Check sheet for the modelled part. Datum: model origin and axes. Units: mm. A direction names the side the tool comes from. Round coordinates to 2 decimals unless told otherwise and drop trailing zeros. Loops run counter-clockwise (first coordinate to the right, second up) from the corner with the lowest first, then second, coordinate; pieces in that order, holes last. Notation, with made-up numbers: M 14,-10 L 55,-10 A9 cw 55,-6 Z; hole C -36.75,-10 d2. An arc over 180 degrees is marked long. One line per question, with ' | ' between items. Start each with the question number.
(1) Section check C-C (z = -23). Record the boundary of the cut face in (x, y), and give its area (3 significant figures).
(2) Section check D-D (y = 37.5). Record the boundary of the cut face in (x, z).
(3) Tool access check on faces 1 (the face through (56, 3, -14)), 2 (the face through (15, 13, -28)), 3 (the face through (34, 0.9, -34)), 4 (the face through (21, 21, -14)), 5 (the face through (59, 1.5, -14)). Record the directions out of +Z, -Z, +X, -X, +Y, -Y that give a thin tool (end or side, any length) a straight path to the whole face; none if there is none.
(4) Draft check along X on faces 6 (the face through (15, 13, 0)), 7 (the face through (0, 2.2, -14.3)), 8 (the face through (66, 4, -14)). Enter one of: +X half, -X half, draft (parallel to the pull), parting line (faces both ways), or undercut.
(5) Go/stop test with flat-tipped pins: P1, Ø8, axis at x = 7.5, y = 11.5, coming from the -Z side; P2, Ø1.5, axis at x = 13, z = -9.5, coming from the +Y side; P3, Ø2, axis at x = 59.5, z = -14, coming from the -Y side. Record where each tip stops, or that it passes through.
(6) Section check B-B (x = 28.5). Record the boundary of the cut face in (y, z).
(7) Thickness scan on probe 1 along Z at (x, y) = (15.5, 16); probe 2 along X at (y, z) = (9.5, -6); probe 3 along Y at (x, z) = (33, -34). Record the ranges inside material, lowest first. Write a range as [from, to].
(8) Section check A-A (y = 21.5). Record the boundary of the cut face in (x, z).
```python
from build123d import *

# Parameters (mm, degrees)
SKETCH1_W           = 21
SKETCH1_H           = 28
BOSS_EXTRUDE1_DEPTH = 3
SKETCH2_W           = 21
SKETCH2_H           = 28
BOSS_EXTRUDE2_DEPTH = 37
CUT_EXTRUDE1_REACH  = 55.151
SHELL1_T            = -1
BOSS_EXTRUDE3_DEPTH = 33.5
SKETCH9_W           = 21
SKETCH9_H           = 28
CUT_EXTRUDE2_DEPTH  = 2
SKETCH10_R          = 1
BOSS_EXTRUDE4_DEPTH = 0.5
CUT_EXTRUDE3_REACH  = 59.099
SKETCH11_W          = 2.558101437
SKETCH11_H          = 1.124051106
MIRROR5_START       = -28
MIRROR5_DEPTH       = 28
MIRROR5_START_2     = 1.5
MIRROR5_2_OUTLINE_R = 1
MIRROR5_2_DEPTH     = 0.5
SHELL3_START        = -27
SHELL3_DEPTH        = 26


# Read off the part's stored shape, not the designer's step: Mirror5, Shell3
with BuildPart() as part:
    # Sketch1 → Boss-Extrude1 (new body)
    with BuildSketch(Plane(origin=(0, 0, 0), x_dir=(1, 0, 0), z_dir=(0, 1, 0))):
        with Locations((10.5, 14)):
            Rectangle(SKETCH1_W, SKETCH1_H)
    extrude(amount=BOSS_EXTRUDE1_DEPTH)

    # Sketch2 → Boss-Extrude2 (add)
    with BuildSketch(Plane(origin=(0, 3, 0), x_dir=(1, 0, 0), z_dir=(0, 1, 0))):
        with Locations((10.5, 14)):
            Rectangle(SKETCH2_W, SKETCH2_H)
    extrude(amount=BOSS_EXTRUDE2_DEPTH)

    # Sketch3 → Cut-Extrude1 (cut, up to next)
    with BuildSketch(Plane.XY, mode=Mode.PRIVATE) as cut_extrude1_sk1:
        Polygon((0, 3), (21, 40), (0, 40), align=None)
    cut_extrude1_tool1 = extrude(cut_extrude1_sk1.sketch, amount=-CUT_EXTRUDE1_REACH, mode=Mode.PRIVATE) & part.part
    add(cut_extrude1_tool1.solids().sort_by_distance((7, 27.666667, 0))[0], mode=Mode.SUBTRACT)

    # Shell1
    shell1_openings = [part.faces().sort_by_distance(p)[0] for p in [
        (10.5, 21.5, -14),
    ]]
    offset(amount=SHELL1_T, openings=shell1_openings, kind=Kind.INTERSECTION)

    # Sketch7 → Boss-Extrude3 (add)
    with BuildSketch(Plane(origin=(0, 0, 0), x_dir=(0, 0, -1), z_dir=(1, 0, 0))):
        Polygon((34, -0.1), (32.967936428, -0.1), (32.967936428, 0.9), (34.5, 0.9), (34.5, 2), (29.5, 2), (-1.5, 2), (-6.5, 2), (-6.5, 0.9), (-4.967936428, 0.9), (-4.967936428, -0.1), (-6, -0.1), (-7.5, -0.1), (-7.5, 3), (-1.5, 3), (29.5, 3), (35.5, 3), (35.5, -0.1), align=None)
    boss_extrude3 = extrude(amount=BOSS_EXTRUDE3_DEPTH)

    # Sketch9 → Cut-Extrude2 (cut)
    with BuildSketch(Plane.XZ):
        with Locations((10.5, -14)):
            Rectangle(SKETCH9_W, SKETCH9_H)
    extrude(amount=-CUT_EXTRUDE2_DEPTH, mode=Mode.SUBTRACT)

    # Sketch10 → Boss-Extrude4 (add)
    with BuildSketch(Plane.XZ.offset(-2)):
        with Locations(Location((8, -14, 0), (0, 0, 90))):
            Circle(SKETCH10_R)
    extrude(amount=BOSS_EXTRUDE4_DEPTH)

    # Sketch11 → Cut-Extrude3 (cut, up to next)
    with BuildSketch(Plane.ZY.offset(-20), mode=Mode.PRIVATE) as cut_extrude3_sk1:
        with Locations((-15.279050719, 10.379008518)):
            Rectangle(SKETCH11_W, SKETCH11_H)
    cut_extrude3_tool1 = extrude(cut_extrude3_sk1.sketch, amount=-CUT_EXTRUDE3_REACH, mode=Mode.PRIVATE) & part.part
    cut_extrude3 = cut_extrude3_tool1.solids().sort_by_distance((20, 10.379009, -15.279051))[0]
    add(cut_extrude3, mode=Mode.SUBTRACT)

    # Mirror4: Boss-Extrude3 across plane
    add(boss_extrude3.mirror(Plane(origin=(33.5, 0, 0), x_dir=(0, 0, 1), z_dir=(1, 0, 0))))

    # Mirror5 outline → Mirror5 (add)
    with BuildSketch(Plane.XY.offset(MIRROR5_START)):
        Polygon((67, 3), (46, 40), (46, 3), align=None)
    extrude(amount=MIRROR5_DEPTH)

    # Mirror5 2 outline → Mirror5 2 (add)
    with BuildSketch(Plane(origin=(0, 0, 0), x_dir=(1, 0, 0), z_dir=(0, 1, 0)).offset(MIRROR5_START_2)):
        with Locations((59, 14)):
            Circle(MIRROR5_2_OUTLINE_R)
    extrude(amount=MIRROR5_2_DEPTH)

    # Shell3 outline → Shell3 (cut)
    with BuildSketch(Plane.XY.offset(SHELL3_START)):
        Polygon((47, 3), (66, 3), (66, 4.761904762), (47, 38.238095238), align=None)
    extrude(amount=SHELL3_DEPTH, mode=Mode.SUBTRACT)

    # Mirror6: Cut-Extrude3 across plane
    add(cut_extrude3.mirror(Plane(origin=(33.5, 0, 0), x_dir=(0, 0, 1), z_dir=(1, 0, 0))), mode=Mode.SUBTRACT)


solid = part.part
```
The answers:
1) outline: M 0,2 L 67,2 L 67,3 L 66,4.76 L 66,3 L 47,3 L 47,38.24 L 46,40 L 46,3 L 21,3 L 21,40 L 20,38.24 L 20,3 L 1,3 L 1,4.76 L 0,3 Z | area: 141 mm²
2) outline: M 19.58,-28 L 21,-28 L 21,0 L 19.58,0 L 19.58,-1 L 20,-1 L 20,-27 L 19.58,-27 Z; M 46,-28 L 47.42,-28 L 47.42,-27 L 47,-27 L 47,-1 L 47.42,-1 L 47.42,0 L 46,0 Z
3) face 1: +Y | face 2: -Z, +X, -X, +Y | face 3: +X, -X | face 4: +Z, -Z, +Y | face 5: +X, -X, -Y
4) face 6: draft | face 7: -X half | face 8: undercut
5) P1: z = -28 | P2: y = 3 | P3: y = 1.5
6) outline: M -0.1,-35.5 L 3,-35.5 L 3,7.5 L -0.1,7.5 L -0.1,4.97 L 0.9,4.97 L 0.9,6.5 L 2,6.5 L 2,-34.5 L 0.9,-34.5 L 0.9,-32.97 L -0.1,-32.97 Z
7) probe 1: [-28, -27], [-1, 0] | probe 2: [20, 21], [46, 47] | probe 3: [-0.1, 0.9], [2, 3]
8) outline: M 10.5,-28 L 21,-28 L 21,0 L 10.5,0 L 10.5,-1 L 20,-1 L 20,-27 L 10.5,-27 Z; M 46,-28 L 56.5,-28 L 56.5,-27 L 47,-27 L 47,-1 L 56.5,-1 L 56.5,0 L 46,0 Z
